Autodesk Inventor part; units mm, degrees
ref_plane "YZ Plane" through (0, 0, 0) normal (1, 0, 0) x (0, 1, 0)
ref_plane "XZ Plane" through (0, 0, 0) normal (0, 1, 0) x (-1, 0, 0)
ref_plane "XY Plane" through (0, 0, 0) normal (0, 0, 1) x (1, 0, 0)
sketch "Sketch1" plane through (0, 0, 0) normal (0, 0, 1) x (1, 0, 0)
  arc A0 (9.3, -7.8) -> (7.8, -9.3) centre (9.3, -9.3) ccw
  line L0 (13.5, -7.8) -> (9.3, -7.8)
  arc A1 (14, -8.3) -> (13.5, -7.8) centre (13.5, -8.3) ccw
  line L1 (14, -12.5) -> (14, -8.3)
  arc A2 (12.5, -14) -> (14, -12.5) centre (12.5, -12.5) ccw
  line L2 (8.3, -14) -> (12.5, -14)
  arc A3 (7.8, -13.5) -> (8.3, -14) centre (8.3, -13.5) ccw
  line L3 (7.8, -9.3) -> (7.8, -13.5)
  arc A4 (-13.5, -7.8) -> (-14, -8.3) centre (-13.5, -8.3) ccw
  line L4 (-9.3, -7.8) -> (-13.5, -7.8)
  arc A5 (-7.8, -9.3) -> (-9.3, -7.8) centre (-9.3, -9.3) ccw
  line L5 (-7.8, -13.5) -> (-7.8, -9.3)
  arc A6 (-8.3, -14) -> (-7.8, -13.5) centre (-8.3, -13.5) ccw
  line L6 (-12.5, -14) -> (-8.3, -14)
  arc A7 (-14, -12.5) -> (-12.5, -14) centre (-12.5, -12.5) ccw
  line L7 (-14, -8.3) -> (-14, -12.5)
  line L8 (3.2859, 3.8789) -> (2.2431, 3.6573)
  arc A8 (3.8789, 3.2859) -> (3.2859, 3.8789) centre (3.3898, 3.3898) ccw
  line L9 (3.6573, 2.2431) -> (3.8789, 3.2859)
  line L10 (3.2627, 1.8485) -> (3.6573, 2.2431)
  line L11 (3.6573, -2.2431) -> (3.2627, -1.8485)
  line L12 (3.8789, -3.2859) -> (3.6573, -2.2431)
  arc A9 (3.2859, -3.8789) -> (3.8789, -3.2859) centre (3.3898, -3.3898) ccw
  line L13 (2.2431, -3.6573) -> (3.2859, -3.8789)
  line L14 (1.8485, -3.2627) -> (2.2431, -3.6573)
  arc A10 (-1.8485, -3.2627) -> (1.6602, -3.3625) centre (0, 0) ccw
  line L15 (-2.2431, -3.6573) -> (-1.8485, -3.2627)
  line L16 (-3.2859, -3.8789) -> (-2.2431, -3.6573)
  arc A11 (-3.8789, -3.2859) -> (-3.2859, -3.8789) centre (-3.3898, -3.3898) ccw
  line L17 (-3.6573, -2.2431) -> (-3.8789, -3.2859)
  line L18 (-3.2627, -1.8485) -> (-3.6573, -2.2431)
  arc A12 (-3.3625, 1.6602) -> (-3.2627, -1.8485) centre (0, 0) ccw
  line L19 (-3.6573, 2.2431) -> (-3.2627, 1.8485)
  line L20 (-3.8789, 3.2859) -> (-3.6573, 2.2431)
  arc A13 (-3.2859, 3.8789) -> (-3.8789, 3.2859) centre (-3.3898, 3.3898) ccw
  line L21 (-2.2431, 3.6573) -> (-3.2859, 3.8789)
  line L22 (-1.8485, 3.2627) -> (-2.2431, 3.6573)
  line L23 (2.2431, 3.6573) -> (1.8485, 3.2627)
  arc A14 (13.5, 7.8) -> (14, 8.3) centre (13.5, 8.3) ccw
  line L24 (9.3, 7.8) -> (13.5, 7.8)
  arc A15 (7.8, 9.3) -> (9.3, 7.8) centre (9.3, 9.3) ccw
  line L25 (7.8, 13.5) -> (7.8, 9.3)
  arc A16 (8.3, 14) -> (7.8, 13.5) centre (8.3, 13.5) ccw
  line L26 (12.5, 14) -> (8.3, 14)
  arc A17 (14, 12.5) -> (12.5, 14) centre (12.5, 12.5) ccw
  line L27 (14, 8.3) -> (14, 12.5)
  arc A18 (-12.5, 14) -> (-14, 12.5) centre (-12.5, 12.5) ccw
  line L28 (-8.3, 14) -> (-12.5, 14)
  arc A19 (-7.8, 13.5) -> (-8.3, 14) centre (-8.3, 13.5) ccw
  line L29 (-7.8, 9.3) -> (-7.8, 13.5)
  arc A20 (-9.3, 7.8) -> (-7.8, 9.3) centre (-9.3, 9.3) ccw
  line L30 (-13.5, 7.8) -> (-9.3, 7.8)
  arc A21 (-14, 8.3) -> (-13.5, 7.8) centre (-13.5, 8.3) ccw
  line L31 (-14, 12.5) -> (-14, 8.3)
  line L32 (12.5, 4.1) -> (12.5, 6.8)
  line L33 (15, 4.1) -> (12.5, 4.1)
  line L34 (15, 15) -> (15, 4.1)
  line L35 (4.1, 15) -> (15, 15)
  line L36 (4.1, 12.5) -> (4.1, 15)
  line L37 (6.8, 12.5) -> (4.1, 12.5)
  line L38 (6.8, 7.8606) -> (6.8, 12.5)
  line L39 (3.9715, 5.0321) -> (6.8, 7.8606)
  line L40 (-3.9715, 5.0321) -> (3.9715, 5.0321)
  line L41 (-6.8, 7.8606) -> (-3.9715, 5.0321)
  line L42 (-6.8, 12.5) -> (-6.8, 7.8606)
  line L43 (-4.1, 12.5) -> (-6.8, 12.5)
  line L44 (-4.1, 15) -> (-4.1, 12.5)
  line L45 (-15, 15) -> (-4.1, 15)
  line L46 (-15, 4.1) -> (-15, 15)
  line L47 (-12.5, 4.1) -> (-15, 4.1)
  line L48 (-12.5, 6.8) -> (-12.5, 4.1)
  line L49 (-7.8606, 6.8) -> (-12.5, 6.8)
  line L50 (-5.0321, 3.9715) -> (-7.8606, 6.8)
  line L51 (-5.0321, -3.9715) -> (-5.0321, 3.9715)
  line L52 (-7.8606, -6.8) -> (-5.0321, -3.9715)
  line L53 (-12.5, -6.8) -> (-7.8606, -6.8)
  line L54 (-12.5, -4.1) -> (-12.5, -6.8)
  line L55 (-15, -4.1) -> (-12.5, -4.1)
  line L56 (-15, -15) -> (-15, -4.1)
  line L57 (-4.1, -15) -> (-15, -15)
  line L58 (-4.1, -12.5) -> (-4.1, -15)
  line L59 (-6.8, -12.5) -> (-4.1, -12.5)
  line L60 (-6.8, -7.8606) -> (-6.8, -12.5)
  line L61 (-3.9715, -5.0321) -> (-6.8, -7.8606)
  line L62 (3.9715, -5.0321) -> (-3.9715, -5.0321)
  line L63 (6.8, -7.8606) -> (3.9715, -5.0321)
  line L64 (6.8, -12.5) -> (6.8, -7.8606)
  line L65 (4.1, -12.5) -> (6.8, -12.5)
  line L66 (4.1, -15) -> (4.1, -12.5)
  line L67 (15, -15) -> (4.1, -15)
  line L68 (15, -4.1) -> (15, -15)
  line L69 (12.5, -4.1) -> (15, -4.1)
  line L70 (12.5, -6.8) -> (12.5, -4.1)
  line L71 (7.8606, -6.8) -> (12.5, -6.8)
  line L72 (5.0321, -3.9715) -> (7.8606, -6.8)
  line L73 (5.0321, 3.9715) -> (5.0321, -3.9715)
  line L74 (7.8606, 6.8) -> (5.0321, 3.9715)
  line L75 (12.5, 6.8) -> (7.8606, 6.8)
  arc A22 (-3.2627, 1.8485) -> (-3.3625, 1.6602) centre (0, 0) ccw
  arc A23 (3.3625, 1.6602) -> (3.2627, 1.8485) centre (0, 0) ccw
  arc A24 (1.8485, 3.2627) -> (-1.8485, 3.2627) centre (0, 0) ccw
  arc A25 (1.6602, -3.3625) -> (1.8485, -3.2627) centre (0, 0) ccw
  arc A26 (3.2627, -1.8485) -> (3.3625, 1.6602) centre (0, 0) ccw
extrude "Extrusion1" add sketch "Sketch1" along normal blind 1000
properties part number "30x30-01" material "Aluminum-6061"
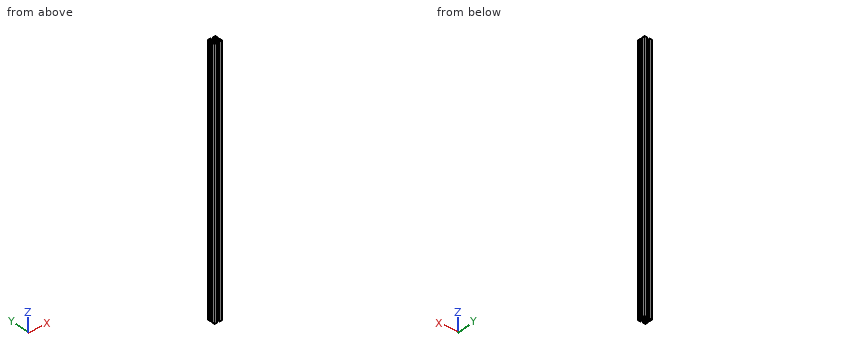
Read the model definition and answer for the solid it produces. Units are mm, in the model's axes. Give positions to 0.01 mm unless a question says otherwise; leave off trailing zeros. One line per item, written item: value. Start each with the question number.
(1) A flat-ended cylindrical pin translates along its axis: pin 1 Ø4 at (x, z) = (1, 575) entering from -Y. Find the tip coordinate at first contact, or state that the pin passes through.
(2) Find section A-A (z = 260). Give the number of separate pieces and of enclosed holes in the cut face, plus the area to 3 significant figures.
(3) Find the intervals of material crossed by line 1 (X direction, y = -13, z = 233); line 2 (Y direction, x = -8.5, z = 634.5); line 3 (Y direction, x = 11, z = 723), in increasing order.
Results below:
1. pin 1: stops at y = -5.03
2. separate pieces: 1
2. enclosed holes: 5
2. area: 241 mm^2
3. line 1: x = -15 to -13.91, -7.8 to -4.1, 4.1 to 7.8, 13.91 to 15
3. line 2: y = -15 to -14, -8.03 to -6.8, 6.8 to 8.03, 14 to 15
3. line 3: y = -15 to -14, -7.8 to -6.8, 6.8 to 7.8, 14 to 15
